Can you work these out from the model? Positions are in its coordinate system, mm. A direction names the side the tool comes from. Give positions to 0.01 mm unless a question says otherwise; leave off trailing zeros. Loops run counter-clockwise (first coordinate to the right, second up) from the corner with the lowest first, then second, coordinate; pieces in that order, holes last. Notation, with made-up numbers: (85, 58) - (99, 58) arc R23 cw to (99, 80) - close; hole circle Ø4 at (42, 39.25). An arc over 180 degrees is marked (long way). Use a Markdown table: item, result. Add a question column.
```python
from build123d import *

# Parameters (mm, degrees)
CROQUIS1_R              = 10
SALIENTE_EXTRUIR2_DEPTH = 50
CROQUIS4_R              = 25
SALIENTE_EXTRUIR3_DEPTH = 3
SALIENTE_EXTRUIR4_START = 25
CROQUIS5_R              = 25
SALIENTE_EXTRUIR4_DEPTH = 3
REDONDEO2_R             = 10
CORTAR_EXTRUIR1_START   = 50
CORTAR_EXTRUIR1_DEPTH   = 20
CORTAR_EXTRUIR2_START   = 50
CROQUIS7_W              = 3.5
CROQUIS7_H              = 7.2
CORTAR_EXTRUIR2_DEPTH   = 10
CORTAR_EXTRUIR3_START   = 1.785357468
CORTAR_EXTRUIR3_DEPTH   = 8.214642632
CORTAR_EXTRUIR4_START   = 24.165153
CROQUIS9_R              = 2
CORTAR_EXTRUIR4_DEPTH   = 3.834847


# Read off the part's stored shape, not the designer's step: Cortar-Extruir3
with BuildPart() as part:
    # Croquis1 → Saliente-Extruir2 (new body)
    with BuildSketch(Plane.XY):
        Circle(CROQUIS1_R)
    extrude(amount=SALIENTE_EXTRUIR2_DEPTH)

    # Croquis4 → Saliente-Extruir3 (add)
    with BuildSketch(Plane.XY):
        Circle(CROQUIS4_R)
    extrude(amount=SALIENTE_EXTRUIR3_DEPTH)

    # Croquis5 → Saliente-Extruir4 (add)
    with BuildSketch(Plane.XY.offset(SALIENTE_EXTRUIR4_START)):
        Circle(CROQUIS5_R)
    extrude(amount=SALIENTE_EXTRUIR4_DEPTH)

    # Redondeo2
    redondeo2_edges = [part.edges().sort_by_distance(p)[0] for p in [
        (-10, 0, 25),
        (-10, 0, 3),
    ]]
    fillet(redondeo2_edges, radius=REDONDEO2_R)

    # Croquis6 → Cortar-Extruir1 (cut)
    with BuildSketch(Plane.XY.offset(CORTAR_EXTRUIR1_START)):
        with BuildLine():
            Line((2, 1.5), (2, -1.5))
            ThreePointArc((2, -1.5), (-2.5, 0), (2, 1.5))
        make_face()
    extrude(amount=-CORTAR_EXTRUIR1_DEPTH, mode=Mode.SUBTRACT)

    # Croquis7 → Cortar-Extruir2 (cut)
    with BuildSketch(Plane.XY.offset(CORTAR_EXTRUIR2_START)):
        with Locations((5.5, 0)):
            Rectangle(CROQUIS7_W, CROQUIS7_H)
    extrude(amount=-CORTAR_EXTRUIR2_DEPTH, mode=Mode.SUBTRACT)

    # Cortar-Extruir3 outline → Cortar-Extruir3 (cut)
    with BuildSketch(Plane(origin=(0, 0, 0), x_dir=(0, 0, -1), z_dir=(1, 0, 0)).offset(CORTAR_EXTRUIR3_START)):
        with BuildLine():
            add(Edge.make_bspline(
                [(-43.250000008, 0), (-43.250010298, 0.457042806), (-43.439269311, 0.91355666), (-44.08377392, 1.559232298), (-44.536167579, 1.749638189), (-45.461098225, 1.750360744), (-45.914256169, 1.560125471), (-46.558728463, 0.916635921), (-46.75, 0.463408547), (-46.75, -0.463408547), (-46.559497121, -0.915462774), (-45.915045576, -1.559741953), (-45.458501244, -1.749734355), (-44.543528816, -1.750265056), (-44.088756623, -1.563446648), (-43.437067231, -0.912124478), (-43.250180582, -0.457964068), (-43.250000045, -0.000460382), (-43.250000003, -0.000230191), (-43.250000008, 0)],
                knots=[0.500062925, 0.500062925, 0.500062925, 0.500062925, 0.625, 0.625, 0.750000001, 0.750000001, 0.875000002, 0.875000002, 1.000000004, 1.000000004, 1.125000006, 1.125000006, 1.250000009, 1.250000009, 1.375000013, 1.375000013, 1.500000015, 1.500000015, 1.50006294, 1.50006294, 1.50006294, 1.50006294], degree=3))
        make_face()
    extrude(amount=CORTAR_EXTRUIR3_DEPTH, mode=Mode.SUBTRACT)

    # Croquis9 → Cortar-Extruir4 (cut)
    with BuildSketch(Plane.XY.offset(CORTAR_EXTRUIR4_START)):
        with Locations((18, 0)):
            Circle(CROQUIS9_R)
    extrude(amount=CORTAR_EXTRUIR4_DEPTH, mode=Mode.SUBTRACT)


solid = part.part
```
1. Suppose I cut it at D-D (z = 18). List the corners of the cut face in (x, y) for me.
2. On a 3-axis mill with a long thin cutter (end or side, diameter ignored), from which of +Z, -Z, +X, -X, +Y, -Y can I reach the whole of each face in a straight line? I mean faces 1 (the face through (0, 0, 0)), 2 (the face through (-2.17, -9.76, 38.85)), 3 (the face through (-11, 17, 25)). Say none if no direction works.
3. Suppose I cut it at B-B (z = 31.5). List the corners of the cut face in (x, y) for me, and give its area (3 significant figures).
4. Please list where these lines run through material, in increasing order: line 1 along Z through (x, y) = (-10, -21.5); line 2 along X through (y, z) = (0, 34.5); line 3 along Y through (x, z) = (0, 35). Write a range as [from, to].
5. Will these pins go through, and if not, where does the flat tip stop? P1, Ø1, axis at x = 5.5, z = 47, coming from the +Y side; P2, Ø3.5, axis at x = 18, y = 0, coming from the +Z side; P3, Ø1, axis at x = 6, y = -0.5, coming from the +Z side.
6. If we mould it in two halves opening along Y, with no side actions, what happens to faces 4 (the face through (0, 0, 30)), 5 (the face through (-2, -2, 50)), 6 (the face through (23.846, 7.509, 1.479)), 7 (the face through (16, 0, 26))? For each: released by +Y, released by -Y, zero draft, split by the parting line, or undercut.
7. Suppose I cut it at C-C (x = 18). State how many separate pieces and enclosed holes the cut face has, and give its area (3 significant figures).
8. Suppose I cut it at A-A (x = 0). List the corners of the cut face in (y, z) for me.
Results below:
| question | item | result |
|---|---|---|
| 1 | outline | circle Ø20.92 at (0, 0) |
| 2 | face 1 | -Z, +X, -X, +Y, -Y |
| 2 | face 2 | +Z |
| 2 | face 3 | none |
| 3 | outline | circle Ø20 at (0, 0); hole (2, -1.5) - (2, 1.5) arc R2.5 ccw (long way) to start |
| 3 | area | 296 mm² |
| 4 | line 1 | [0, 3], [25, 28] |
| 4 | line 2 | [-10, -2.5], [2, 10] |
| 4 | line 3 | [-10, -2.5], [2.5, 10] |
| 5 | P1 | y = 8.66 |
| 5 | P2 | z = 3.73 |
| 5 | P3 | z = 40 |
| 6 | face 4 | undercut |
| 6 | face 5 | zero draft |
| 6 | face 6 | split by the parting line |
| 6 | face 7 | undercut |
| 7 | separate pieces | 3 |
| 7 | enclosed holes | 0 |
| 7 | area | 199 mm² |
| 8 | outline | (-25, 0) - (25, 0) - (25, 3) - (20, 3) arc R10 cw to (10, 13) - (10, 15) arc R10 cw to (20, 25) - (25, 25) - (25, 28) - (10, 28) - (10, 50) - (2.5, 50) - (2.5, 30) - (-2.5, 30) - (-2.5, 50) - (-10, 50) - (-10, 28) - (-25, 28) - (-25, 25) - (-20, 25) arc R10 cw to (-10, 15) - (-10, 13) arc R10 cw to (-20, 3) - (-25, 3) - close |
